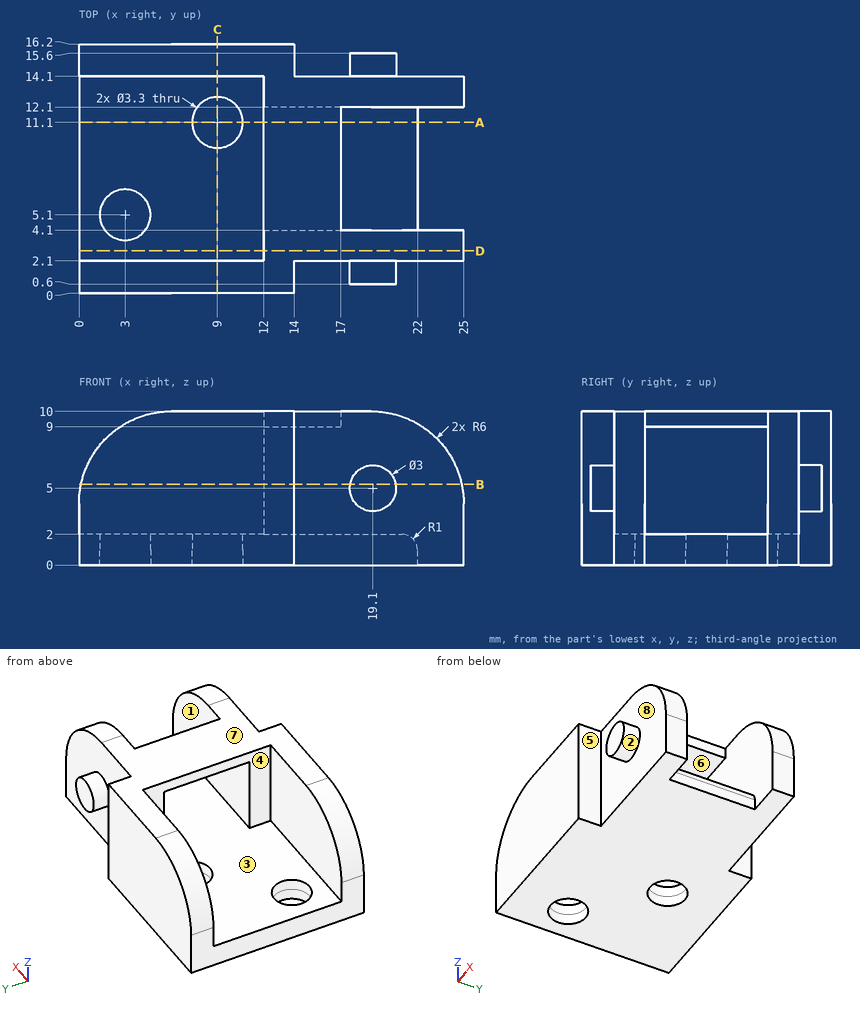
The figure shows three views and two pictorial views of one solid part (mm, origin at its lowest corner). Answer the questions. A direction names the side the tool comes from. Coordinates: 2 decimals unless noted, no trailing zeros. Loops run counter-clockwise (first coordinate to the right, second up) from the corner with the lowest first, then second, coordinate; pieces in that order, holes last. Notation, with made-up numbers: (66.25, 53.25) - (81.25, 53.25) arc R17 cw to (81.25, 86.25) - close; hole circle Ø5 at (56.5, 4). An arc over 180 degrees is marked (long way). Write item = value, one per line.
1) Section A-A (y = 11.1) is taken. Determine the outline of the cut face in (x, z), plus the area to 3 significant figures.
Responses:
outline = (0, 0) - (7.35, 0) - (7.35, 2) - (0, 2) - close; (10.65, 0) - (22, 0) - (22, 1) arc R1 ccw to (21, 2) - (10.65, 2) - close; (12, 9) - (17, 9) - (17, 10) - (12, 10) - close
area = 42.2 mm^2
2) Determine the mould class of the marked faces 6, 7 and 8 for opening direction Z: pulls with the +Z half, pulls with the -Z half, needs draft (parallel to the pull), parting line crosses it, or undercut.
Responses:
face_6 = undercut
face_7 = pulls with the +Z half
face_8 = needs draft
3) Find the intervals of material crossed by line 1 along Z through (x, y) = (16.75, 9.75); line 2 along Y through (x, z) = (9.75, 6.25); line 3 along Y through (x, z) = (3, 0.65), in increasing order.
Responses:
line_1 = 0 to 2, 9 to 10
line_2 = 0 to 2.1, 14.1 to 16.2
line_3 = 0 to 3.45, 6.75 to 16.2
4) Section B-B (z = 5.25) is taken. Determine the outline of the cut face in (x, y), plus the area to 3 significant figures.
Responses:
outline = (0.13, 0) - (14, 0) - (14, 2.1) - (17.62, 2.1) - (17.62, 0.6) - (20.58, 0.6) - (20.58, 2.1) - (24.87, 2.1) - (24.87, 4.1) - (12, 4.1) - (12, 2.1) - (0.13, 2.1) - close; (0.13, 14.1) - (12, 14.1) - (12, 12.1) - (24.87, 12.1) - (24.87, 14.1) - (20.58, 14.1) - (20.58, 15.6) - (17.62, 15.6) - (17.62, 14.1) - (14, 14.1) - (14, 16.2) - (0.13, 16.2) - close
area = 119 mm^2
5) Section C-C (x = 9) is taken. Determine the outline of the cut face in (y, z), plus the area to 3 significant figures.
Responses:
outline = (0, 0) - (9.45, 0) - (9.45, 2) - (2.1, 2) - (2.1, 10) - (0, 10) - close; (12.75, 0) - (16.2, 0) - (16.2, 10) - (14.1, 10) - (14.1, 2) - (12.75, 2) - close
area = 59.4 mm^2
6) Which of the six approach directions +Z, -Z, +X, -X, +Y, -Y give full straight-line access (tool end or side, diameter ignored) to the marked faces 1, 2, 3, 4 and 5?
Responses:
face_1 = +X
face_2 = -Y
face_3 = -X
face_4 = +Z, -X
face_5 = +Z, -Z, -Y
7) Section D-D (y = 2.75) is taken. Determine the outline of the cut face in (x, z).
Responses:
outline = (0, 0) - (25, 0) - (25, 4) arc R6 ccw to (19, 10) - (12, 10) - (12, 2) - (0, 2) - close
8) Each of these flat-tipped pins is pushed along its axis until it touches: P1, Ø5.5, axis at x = 3, y = 5.1, coming from the +Z side; P2, Ø0.8, axis at y = 8.5, z = 9.5, coming from the +X side; P3, Ø0.6, axis at y = 1.5, z = 3, coming from the +X side; P4, Ø3, axis at x = 9, y = 11.1, coming from the +Z side. Where does it stop, or does it pass through?
Responses:
P1 = 2
P2 = 17
P3 = 14
P4 = through
